from build123d import *

# Parameters (mm, degrees)
SKETCH1_W           = 42
SKETCH1_H           = 42
BOSS_EXTRUDE1_DEPTH = 47
CHAMFER1_SIZE       = 4
BOSS_EXTRUDE4_DEPTH = 5
BOSS_EXTRUDE5_DEPTH = 5
SKETCH2_R           = 16.25
CUT_EXTRUDE1_DEPTH  = 0.4
SKETCH3_R           = 11
SKETCH3_R_2         = 4
BOSS_EXTRUDE2_DEPTH = 1.9
SKETCH4_R           = 2.5
BOSS_EXTRUDE3_DEPTH = 23
CHAMFER2_SIZE       = 0.5
SKETCH5_R           = 1.5
CUT_EXTRUDE2_DEPTH  = 5
SKETCH8_W           = 4.8
SKETCH8_H           = 3.8
SKETCH8_W_2         = 4.5
SKETCH8_H_2         = 3.5
BOSS_EXTRUDE6_DEPTH = 0.1


with BuildPart() as part:
    # Sketch1 → Boss-Extrude1 (new body)
    with BuildSketch(Plane(origin=(0, 0, 0), x_dir=(1, 0, 0), z_dir=(0, 1, 0))):
        Rectangle(SKETCH1_W, SKETCH1_H)
    extrude(amount=BOSS_EXTRUDE1_DEPTH)

    # Chamfer1
    chamfer1_edges = [part.edges().sort_by_distance(p)[0] for p in [
        (21, 23.5, 21),
        (-21, 23.5, 21),
        (-21, 23.5, -21),
        (21, 23.5, -21),
    ]]
    chamfer(chamfer1_edges, length=CHAMFER1_SIZE)

    # Sketch6 → Boss-Extrude4 (add)
    with BuildSketch(Plane(origin=(0, 47, 0), x_dir=(1, 0, 0), z_dir=(0, 1, 0))):
        Polygon((17.062132034, 21.15), (-17.062132034, 21.15), (-21.15, 17.062132034), (-21.15, -17.062132034), (-17.062132034, -21.15), (17.062132034, -21.15), (21.15, -17.062132034), (21.15, 17.062132034), align=None)
    extrude(amount=-BOSS_EXTRUDE4_DEPTH)

    # Sketch7 → Boss-Extrude5 (add)
    with BuildSketch(Plane.XZ):
        Polygon((-21.15, 17.062132034), (-21.15, -17.062132034), (-17.062132034, -21.15), (17.062132034, -21.15), (21.15, -17.062132034), (21.15, 17.062132034), (17.062132034, 21.15), (-17.062132034, 21.15), align=None)
    extrude(amount=-BOSS_EXTRUDE5_DEPTH)

    # Sketch2 → Cut-Extrude1 (cut)
    with BuildSketch(Plane(origin=(0, 47, 0), x_dir=(1, 0, 0), z_dir=(0, 1, 0))):
        with Locations(Location((0, 0, 0), (0, 0, 270))):
            Circle(SKETCH2_R)
    extrude(amount=-CUT_EXTRUDE1_DEPTH, mode=Mode.SUBTRACT)

    # Sketch3 → Boss-Extrude2 (add)
    with BuildSketch(Plane(origin=(0, 46.6, 0), x_dir=(1, 0, 0), z_dir=(0, 1, 0))):
        with Locations(Location((0, 0, 0), (0, 0, 90))):
            Circle(SKETCH3_R)
        with Locations(Location((0, 0, 0), (0, 0, 90))):
            Circle(SKETCH3_R_2, mode=Mode.SUBTRACT)
    extrude(amount=BOSS_EXTRUDE2_DEPTH)

    # Sketch4 → Boss-Extrude3 (add)
    with BuildSketch(Plane(origin=(0, 46.6, 0), x_dir=(1, 0, 0), z_dir=(0, 1, 0))):
        with Locations(Location((0, 0, 0), (0, 0, 270))):
            Circle(SKETCH4_R)
    extrude(amount=BOSS_EXTRUDE3_DEPTH)

    # Chamfer2
    # the kernel refuses this chamfer: 0.5 mm, written as the material it adds along each edge
    with BuildSketch(Plane(origin=(0, 46.6, 0), x_dir=(0, 0, 1), z_dir=(-1, 0, 0))) as chamfer2_piece_1_section:
        Polygon((16.25, CHAMFER2_SIZE), (16.25 - CHAMFER2_SIZE, 0), (16.25, 0), align=None)
    chamfer2_piece_1 = revolve(axis=Axis((0, 46.6, 0), (0, 1, 0)), mode=Mode.PRIVATE)
    chamfer2_piece_1 = split(chamfer2_piece_1, bisect_by=Plane(origin=(0, 47, -15.959627936), z_dir=(0, -1, 0)), keep=Keep.TOP, mode=Mode.PRIVATE)
    add(chamfer2_piece_1)
    # the kernel refuses this chamfer: 0.5 mm, written as the material it takes off along each edge
    with BuildSketch(Plane(origin=(0, 48.5, 0), x_dir=(0, 0, -1), z_dir=(1, 0, 0))) as chamfer2_2_piece_1:
        Polygon((4 + CHAMFER2_SIZE, 0), (4, -CHAMFER2_SIZE), (4, 0), align=None)
    revolve(axis=Axis((0, 48.5, 0), (0, 1, 0)), mode=Mode.SUBTRACT)
    with BuildSketch(Plane(origin=(0, 48.5, 0), x_dir=(0, 0, -1), z_dir=(1, 0, 0))) as chamfer2_2_piece_2:
        Polygon((11, -CHAMFER2_SIZE), (11 - CHAMFER2_SIZE, 0), (11, 0), align=None)
    revolve(axis=Axis((0, 48.5, 0), (0, 1, 0)), mode=Mode.SUBTRACT)
    with BuildSketch(Plane(origin=(0, 69.6, 0), x_dir=(0, 0, 1), z_dir=(-1, 0, 0))) as chamfer2_2_piece_3:
        Polygon((2.5, -CHAMFER2_SIZE), (2.5 - CHAMFER2_SIZE, 0), (2.5, 0), align=None)
    revolve(axis=Axis((0, 69.6, 0), (0, 1, 0)), mode=Mode.SUBTRACT)

    # Sketch5 → Cut-Extrude2 (cut)
    with BuildSketch(Plane(origin=(0, 47, 0), x_dir=(1, 0, 0), z_dir=(0, 1, 0))):
        with Locations(Location((-15.5, 15.5, 0), (0, 0, 270))):
            Circle(SKETCH5_R)
        with Locations(Location((15.5, 15.5, 0), (0, 0, 270))):
            Circle(SKETCH5_R)
        with Locations(Location((15.5, -15.5, 0), (0, 0, 270))):
            Circle(SKETCH5_R)
        with Locations(Location((-15.5, -15.5, 0), (0, 0, 270))):
            Circle(SKETCH5_R)
    extrude(amount=-CUT_EXTRUDE2_DEPTH, mode=Mode.SUBTRACT)

    # Sketch8 → Boss-Extrude6 (add)
    with BuildSketch(Plane(origin=(21.15, 0, 0), x_dir=(0, 0, -1), z_dir=(1, 0, 0))):
        with Locations((0.269797982, 2.75)):
            Rectangle(SKETCH8_W, SKETCH8_H)
        with Locations((0.269797982, 2.75)):
            Rectangle(SKETCH8_W_2, SKETCH8_H_2, mode=Mode.SUBTRACT)
    extrude(amount=BOSS_EXTRUDE6_DEPTH)


solid = part.part
Verification items for the finished model (mm, model axes). A direction names the side the tool comes from. Give positions to 0.01 mm unless a question says otherwise; leave off trailing zeros. Loops run counter-clockwise (first coordinate to the right, second up) from the corner with the lowest first, then second, coordinate; pieces in that order, holes last.
1. Tool access check on faces 5 (the flat face through (21, 23, 0)), 6 (the flat face through (11, 46.6, 3)), 7 (the flat face through (19.08, 44.54, 19.13)). Record the directions out of +Z, -Z, +X, -X, +Y, -Y that give a thin tool (end or side, any length) a straight path to the whole face; none if there is none.
Derived:
face 5: +Z, -Z, +X
face 6: +Y
face 7: +Z, +X, +Y, -Y
2. Material ranges on probe 1 along X at (y, z) = (47.3, 0); probe 2 along X at (y, z) = (44.55, -15.5); probe 3 along Y at (x, z) = (-2.5, 7.5), recorded low to high.
Derived:
probe 1: x = -11 to -4, -2.5 to 2.5, 4 to 11
probe 2: x = -21.15 to -17, -14 to 14, 17 to 21.15
probe 3: y = 0 to 48.5
3. Go/stop test with flat-tipped pins: P1, Ø8, axis at y = 10.5, z = 15.5, coming from the +X side; P2, Ø12, axis at x = 14.5, y = 27.5, coming from the +Z side; P3, Ø2.5, axis at y = 45.5, z = -2.5, coming from the +X side. Record where each tip stops, or that it passes through.
Derived:
P1: stops at x = 21
P2: stops at z = 21
P3: stops at x = 21.15
4. Cross-section at A-A on y = 56.5. Record the cut outline in (x, z), and give its area (3 significant figures).
Derived:
outline: circle Ø5 at (0, 0)
area: 19.6 mm2
5. Release check for a two-part mould opening along Z. For faces 1 (the cylindrical face through (15.57, 44.54, -17)), 2 (the flat face through (0, 2, 21.15)), 3 (the flat face through (0, 45, -21.15)), 4 (the flat face through (21.15, 45, 0)) record: +Z half, -Z half, draft (parallel to the pull), parting line (faces both ways), or undercut.
Derived:
face 1: undercut
face 2: +Z half
face 3: -Z half
face 4: draft
